Geometry: final body of the model. Coordinates: model frame, mm. A direction names the side the tool comes from. Give positions to 0.01 mm unless a question says otherwise; leave off trailing zeros. Order: outer loops, then holes, each group sorted by start corner. A loop starts at its lowest first (then second) coordinate and runs counter-clockwise, first axis right, second up. Notation, with made-up numbers: (-15.5, 85.25) -> (20.5, 85.25) arc R34 cw to (20.5, 119.25) -> close; hole circle Ø1 at (72, 30.25). An arc over 180 degrees is marked (long way). One line per question, with ' | ' between items. Start each with the question number.
(1) Section B-B (x = 60.5). Return loops of the section in (y, z).
(2) Mould query, pull axis Y, two halves, no side actions, for faces 6 (the face through (57, -23, 2)), 7 (the face through (35, -53, 5)), 8 (the face through (43.6, -91, -44.8)). Classes: +Y half, -Y half, draft (parallel to the pull), parting line (faces both ways), or undercut.
(3) First-contact query: pin 1 Ø1.5 at (x, z) = (46, -25.5) entering from +Y; pin 2 Ø12 at (y, z) = (-73.5, -6.5) entering from -X; pin 3 Ø6.5 at (x, y) = (60.5, -22.94) entering from -Z; pin 4 Ø13 at (x, z) = (40.5, -54) entering from +Y. Flat tips, straight axial feed; report the tip coordinate or a pass-through.
(4) Section D-D (z = -38.5). Return loops of the section in (x, y), then the cut area to 3 significant figures.
(5) Section A-A (z = -21.66). Return loops of the section in (x, y).
(6) Section C-C (y = -50). Return loops of the section in (x, z).
(7) Set-up query: faces 1 (the face through (43, -31.078, -21)), 2 (the face through (42, -27.878, -15)), 3 (the face through (44, -87.575, -54)), 4 (the face through (49.56, -53, -44)), 5 (the face through (43, -51, -46.5)). Return all of +Z, -Z, +X, -X, +Y, -Y with unobstructed straight access to the full face (end or side cutting, diameter ignored); none if empty.
(8) Ray query, L1, parallel to Y at x = 60.5, z = 3.6; L2, parallel to Z at x = 40, y = -69; L3, parallel to X at y = -74.5, z = -45. Return the intervals inside material, ascending.
```python
from build123d import *

# Parameters (mm, degrees)
BOSS_EXTRUDE1_DEPTH   = 5
SKETCH2_W             = 6.35
SKETCH2_H             = 50
BOSS_EXTRUDE2_DEPTH   = 52.48
CUT_EXTRUDE1_REACH    = 106.448
SKETCH3_R             = 20.44
SKETCH3_R_2           = 2.555
SKETCH3_W             = 5
SKETCH3_H             = 50
CUT_EXTRUDE2_REACH    = 108.104
SKETCH4_R             = 3.5
CUT_EXTRUDE6_REACH    = 108.104
SKETCH14_W            = 23.196263878
SKETCH14_H            = 15.316152196
SKETCH15_W            = 12
SKETCH15_H            = 3.2
BOSS_EXTRUDE7_DEPTH   = 46.5
BOSS_EXTRUDE8_REACH   = 98.667
SKETCH16_W            = 12
SKETCH16_H            = 3.5
SKETCH17_W            = 12
SKETCH17_H            = 3.5
BOSS_EXTRUDE9_DEPTH   = 15
CHAMFER2_SIZE         = 2
SKETCH22_W            = 12
SKETCH22_H            = 15
BOSS_EXTRUDE10_DEPTH  = 0.72
CUT_EXTRUDE8_REACH    = 103.606
CUT_EXTRUDE7_REACH    = 120.762
SKETCH18_R            = 3.25
MIRROR2_OUTLINE_W     = 50
MIRROR2_OUTLINE_H     = 5
MIRROR2_DEPTH         = 68
MIRROR2_2_OUTLINE_R   = 2.555
MIRROR2_2_OUTLINE_R_2 = 20.44
MIRROR2_2_DEPTH       = 6.35
MIRROR2_START         = 37.56
MIRROR2_3_DEPTH       = 12
MIRROR2_START_2       = 51
MIRROR2_4_OUTLINE_W   = 13.938985111
MIRROR2_4_OUTLINE_H   = 5
MIRROR2_4_DEPTH       = 5.9999999
MIRROR2_START_3       = 64.0000001
MIRROR2_5_OUTLINE_W   = 13.938985111
MIRROR2_5_OUTLINE_H   = 5
MIRROR2_5_DEPTH       = 5.9999999
MIRROR2_6_DEPTH       = 5
BOSS_EXTRUDE11_DEPTH  = 12
CUT_EXTRUDE9_REACH    = 132.799
SKETCH26_W            = 121.241742099
SKETCH26_H            = 103.992632166


with BuildPart() as part:
    # Sketch1 → Boss-Extrude1 (new body)
    with BuildSketch(Plane.XY):
        Polygon((0, 0), (0, 50), (51, 50), (51, 64.061014889), (70, 64.061014889), (70, -13.938985111), (51, -13.938985111), (51, 0), align=None)
    extrude(amount=BOSS_EXTRUDE1_DEPTH)

    # Sketch2 → Boss-Extrude2 (add)
    with BuildSketch(Plane(origin=(0, 0, 0), x_dir=(-1, 0, 0), z_dir=(0, 0, -1))):
        with Locations((-3.175, 25)):
            Rectangle(SKETCH2_W, SKETCH2_H)
    extrude(amount=BOSS_EXTRUDE2_DEPTH)

    # Sketch3 → Cut-Extrude1 (cut, up to next)
    with BuildSketch(Plane(origin=(6.35, 0, 0), x_dir=(0, 0, -1), z_dir=(1, 0, 0)), mode=Mode.PRIVATE) as cut_extrude1_sk1:
        with Locations((21.66, 25)):
            Circle(SKETCH3_R)
    cut_extrude1_tool1 = extrude(cut_extrude1_sk1.sketch, amount=-CUT_EXTRUDE1_REACH, mode=Mode.PRIVATE) & part.part
    # Sketch3 → Cut-Extrude1 (cut, up to next)
    with BuildSketch(Plane(origin=(6.35, 0, 0), x_dir=(0, 0, -1), z_dir=(1, 0, 0)), mode=Mode.PRIVATE) as cut_extrude1_sk2:
        with Locations((3.695, 42.955)):
            Circle(SKETCH3_R_2)
    cut_extrude1_tool2 = extrude(cut_extrude1_sk2.sketch, amount=-CUT_EXTRUDE1_REACH, mode=Mode.PRIVATE) & part.part
    # Sketch3 → Cut-Extrude1 (cut, up to next)
    with BuildSketch(Plane(origin=(6.35, 0, 0), x_dir=(0, 0, -1), z_dir=(1, 0, 0)), mode=Mode.PRIVATE) as cut_extrude1_sk3:
        with Locations((39.615, 7.045)):
            Circle(SKETCH3_R_2)
    cut_extrude1_tool3 = extrude(cut_extrude1_sk3.sketch, amount=-CUT_EXTRUDE1_REACH, mode=Mode.PRIVATE) & part.part
    # Sketch3 → Cut-Extrude1 (cut, up to next)
    with BuildSketch(Plane(origin=(6.35, 0, 0), x_dir=(0, 0, -1), z_dir=(1, 0, 0)), mode=Mode.PRIVATE) as cut_extrude1_sk4:
        with Locations((49.98, 25)):
            Rectangle(SKETCH3_W, SKETCH3_H)
    cut_extrude1_tool4 = extrude(cut_extrude1_sk4.sketch, amount=-CUT_EXTRUDE1_REACH, mode=Mode.PRIVATE) & part.part
    add(cut_extrude1_tool1.solids().sort_by_distance((6.35, 25, -21.66))[0], mode=Mode.SUBTRACT)
    add(cut_extrude1_tool2.solids().sort_by_distance((6.35, 42.955, -3.695))[0], mode=Mode.SUBTRACT)
    add(cut_extrude1_tool3.solids().sort_by_distance((6.35, 7.045, -39.615))[0], mode=Mode.SUBTRACT)
    add(cut_extrude1_tool4.solids().sort_by_distance((6.35, 25, -49.98))[0], mode=Mode.SUBTRACT)

    # Sketch4 → Cut-Extrude2 (cut, up to next)
    with BuildSketch(Plane(origin=(0, 0, 0), x_dir=(-1, 0, 0), z_dir=(0, 0, -1)), mode=Mode.PRIVATE) as cut_extrude2_sk1:
        with Locations((-60.5, 55.061014889)):
            Circle(SKETCH4_R)
    cut_extrude2_tool1 = extrude(cut_extrude2_sk1.sketch, amount=-CUT_EXTRUDE2_REACH, mode=Mode.PRIVATE) & part.part
    # Sketch4 → Cut-Extrude2 (cut, up to next)
    with BuildSketch(Plane(origin=(0, 0, 0), x_dir=(-1, 0, 0), z_dir=(0, 0, -1)), mode=Mode.PRIVATE) as cut_extrude2_sk2:
        with Locations((-60.5, -4.938985111)):
            Circle(SKETCH4_R)
    cut_extrude2_tool2 = extrude(cut_extrude2_sk2.sketch, amount=-CUT_EXTRUDE2_REACH, mode=Mode.PRIVATE) & part.part
    add(cut_extrude2_tool1.solids().sort_by_distance((60.5, 55.061015, 0))[0], mode=Mode.SUBTRACT)
    add(cut_extrude2_tool2.solids().sort_by_distance((60.5, -4.938985, 0))[0], mode=Mode.SUBTRACT)

    # Sketch14 → Cut-Extrude6 (cut, up to next)
    with BuildSketch(Plane(origin=(0, 0, 0), x_dir=(-1, 0, 0), z_dir=(0, 0, -1)), mode=Mode.PRIVATE) as cut_extrude6_sk1:
        with Locations((-62.598131939, 57.658076098)):
            Rectangle(SKETCH14_W, SKETCH14_H)
    cut_extrude6_tool1 = extrude(cut_extrude6_sk1.sketch, amount=-CUT_EXTRUDE6_REACH, mode=Mode.PRIVATE) & part.part
    add(cut_extrude6_tool1.solids().sort_by_distance((62.598132, 57.658076, 0))[0], mode=Mode.SUBTRACT)

    # Sketch15 → Boss-Extrude7 (add)
    with BuildSketch(Plane(origin=(0, 0, 0), x_dir=(-1, 0, 0), z_dir=(0, 0, -1))):
        with Locations((-43.56, 1.6)):
            Rectangle(SKETCH15_W, SKETCH15_H)
    extrude(amount=BOSS_EXTRUDE7_DEPTH)

    # Boss-Extrude8: up to this plane
    boss_extrude8_end = Plane(origin=(166.832994776, 64.085435133, -66.619565524), z_dir=(-1.1416993347548052e-15, 0.9990256874715413, 0.04413247978546202))
    # Sketch16 → Boss-Extrude8 (add, up to the surface)
    with BuildSketch(Plane(origin=(0, 3.2, 0), x_dir=(1, 0, 0), z_dir=(0, 1, 0)), mode=Mode.PRIVATE) as boss_extrude8_sk1:
        with Locations((43.56, 44.75)):
            Rectangle(SKETCH16_W, SKETCH16_H)
    boss_extrude8_tool1 = split(extrude(boss_extrude8_sk1.sketch, amount=BOSS_EXTRUDE8_REACH, mode=Mode.PRIVATE), bisect_by=boss_extrude8_end, keep=Keep.BOTH, mode=Mode.PRIVATE)
    add(boss_extrude8_tool1.solids().sort_by_distance((43.56, 3.2, -44.75))[0])

    # Sketch17 → Boss-Extrude9 (add)
    with BuildSketch(Plane(origin=(0, 0, -46.5), x_dir=(-1, 0, 0), z_dir=(0, 0, -1))):
        with Locations((-43.56, 61.446642853)):
            Rectangle(SKETCH17_W, SKETCH17_H)
    extrude(amount=BOSS_EXTRUDE9_DEPTH)

    # Chamfer2
    chamfer2_edges = [part.edges().sort_by_distance(p)[0] for p in [
        (3.175, 0, -47.48),
        (3.175, 50, -47.48),
        (70, 50, 2.5),
    ]]
    chamfer(chamfer2_edges, length=CHAMFER2_SIZE)

    # Sketch22 → Boss-Extrude10 (add)
    with BuildSketch(Plane(origin=(0, 63.196642853, 0), x_dir=(1, 0, 0), z_dir=(0, 1, 0))):
        with Locations((43.56, 54)):
            Rectangle(SKETCH22_W, SKETCH22_H)
    extrude(amount=BOSS_EXTRUDE10_DEPTH)

    # Sketch23 → Cut-Extrude8 (cut, up to next)
    with BuildSketch(Plane(origin=(49.56, 0, 0), x_dir=(0, 0, -1), z_dir=(1, 0, 0)), mode=Mode.PRIVATE) as cut_extrude8_sk1:
        Polygon((46.5, 63.916642853), (46.5, 63.196642853), (61.5, 63.916642853), align=None)
    cut_extrude8_tool1 = extrude(cut_extrude8_sk1.sketch, amount=-CUT_EXTRUDE8_REACH, mode=Mode.PRIVATE) & part.part
    add(cut_extrude8_tool1.solids().sort_by_distance((49.56, 63.676643, -51.5))[0], mode=Mode.SUBTRACT)

    # Cut-Extrude7: up to this plane
    cut_extrude7_end = Plane(origin=(-0.001, 63.196642853, -46.5), z_dir=(-2.1659106514416256e-15, -0.9988499868416298, -0.04794479936839813))
    # Sketch18 → Cut-Extrude7 (cut, up to the surface)
    with BuildSketch(Plane.XZ.offset(-59.696642853), mode=Mode.PRIVATE) as cut_extrude7_sk1:
        with Locations(Location((43.56, -52.57, 0), (0, 0, 270))):
            Circle(SKETCH18_R)
    cut_extrude7_tool1 = split(extrude(cut_extrude7_sk1.sketch, amount=-CUT_EXTRUDE7_REACH, mode=Mode.PRIVATE), bisect_by=cut_extrude7_end, keep=Keep.BOTH, mode=Mode.PRIVATE)
    add(cut_extrude7_tool1.solids().sort_by_distance((43.56, 59.696643, -52.57))[0], mode=Mode.SUBTRACT)



with BuildPart() as body_2:
    # Mirror2: read off the stored shape, not the designer's step
    # Mirror2 outline → Mirror2 (new body)
    with BuildSketch(Plane.YZ):
        with Locations((-52.877970222, 2.5)):
            Rectangle(MIRROR2_OUTLINE_W, MIRROR2_OUTLINE_H)
    extrude(amount=MIRROR2_DEPTH)

    # Mirror2 2 outline → Mirror2 2 (add)
    with BuildSketch(Plane.YZ):
        Polygon((-27.877970222, -45.48), (-27.877970222, 0), (-77.877970222, 0), (-77.877970222, -45.48), (-75.877970222, -47.48), (-29.877970222, -47.48), align=None)
        with Locations((-34.922970222, -39.615)):
            Circle(MIRROR2_2_OUTLINE_R, mode=Mode.SUBTRACT)
        with Locations((-70.832970222, -3.695)):
            Circle(MIRROR2_2_OUTLINE_R, mode=Mode.SUBTRACT)
        with Locations((-52.877970222, -21.66)):
            Circle(MIRROR2_2_OUTLINE_R_2, mode=Mode.SUBTRACT)
    extrude(amount=MIRROR2_2_DEPTH)


with BuildPart() as part_1:
    add(part.part)

    add(body_2.part)  # Mirror2 3 merges body 2
    # Mirror2 3 outline → Mirror2 3 (add)
    with BuildSketch(Plane.YZ.offset(MIRROR2_START)):
        Polygon((-31.077970222, -46.5), (0, -46.5), (0, -43), (-27.877970222, -43), (-27.877970222, 0), (-31.077970222, 0), align=None)
    extrude(amount=MIRROR2_3_DEPTH)

    # Mirror2 4 outline → Mirror2 4 (add)
    with BuildSketch(Plane.YZ.offset(MIRROR2_START_2)):
        with Locations((-20.908477667, 2.5)):
            Rectangle(MIRROR2_4_OUTLINE_W, MIRROR2_4_OUTLINE_H)
    extrude(amount=MIRROR2_4_DEPTH)

    # Mirror2 5 outline → Mirror2 5 (add)
    with BuildSketch(Plane.YZ.offset(MIRROR2_START_3)):
        with Locations((-20.908477667, 2.5)):
            Rectangle(MIRROR2_5_OUTLINE_W, MIRROR2_5_OUTLINE_H)
    extrude(amount=MIRROR2_5_DEPTH)

    # Mirror2 6 outline → Mirror2 6 (add)
    with BuildSketch(Plane.XY):
        Polygon((70, -75.877970222), (70, -27.877970222), (68, -27.877970222), (68, -77.877970222), align=None)
        with BuildLine():
            Line((64.0000001, -27.877970222), (64, -22.938985111))
            ThreePointArc((64, -22.938985111), (60.5, -26.438985111), (57, -22.938985111))
            Line((57, -22.938985111), (56.9999999, -27.877970222))
            Line((56.9999999, -27.877970222), (64.0000001, -27.877970222))
        make_face()
        with BuildLine():
            ThreePointArc((57, -22.938985111), (60.5, -19.438985111), (64, -22.938985111))
            Line((64, -22.938985111), (64.0000001, -13.938985111))
            Line((64.0000001, -13.938985111), (56.9999999, -13.938985111))
            Line((56.9999999, -13.938985111), (57, -22.938985111))
        make_face()
    extrude(amount=MIRROR2_6_DEPTH)

    # Sketch25 → Boss-Extrude11 (add)
    with BuildSketch(Plane(origin=(49.56, 0, 0), x_dir=(0, 0, -1), z_dir=(1, 0, 0))):
        Polygon((43, -13.938985111), (46.5, -13.938985111), (46.5, -87.574613075), (61.5, -87.574613075), (61.5, -91.794613075), (46.5, -91.074613075), (43, -90.919998753), (43, -31.077970222), align=None)
    extrude(amount=-BOSS_EXTRUDE11_DEPTH)

    # Cut-Extrude9: up to this face of the body (flat: up to its plane)
    cut_extrude9_end = Plane(part_1.part.faces().sort_by_distance((0, 0.724855186, -20.24))[0])
    # Sketch26 → Cut-Extrude9 (cut, up to the picked face)
    with BuildSketch(Plane(origin=(70, 0, 0), x_dir=(0, 0, -1), z_dir=(1, 0, 0)), mode=Mode.PRIVATE) as cut_extrude9_sk1:
        with Locations((55.62087105, 38.057330972)):
            Rectangle(SKETCH26_W, SKETCH26_H)
    cut_extrude9_tool1 = split(extrude(cut_extrude9_sk1.sketch, amount=-CUT_EXTRUDE9_REACH, mode=Mode.PRIVATE), bisect_by=cut_extrude9_end, keep=Keep.BOTH, mode=Mode.PRIVATE)
    add(cut_extrude9_tool1.solids().sort_by(Axis((70, 38.057331, -55.620871), (-1, 0, 0)))[0], mode=Mode.SUBTRACT)


solid = part_1.part
```
Response:
1) outline: (-77.88, 0) -> (-26.44, 0) -> (-26.44, 5) -> (-77.88, 5) -> close; (-19.44, 0) -> (-13.94, 0) -> (-13.94, 5) -> (-19.44, 5) -> close
2) face 6: undercut | face 7: draft | face 8: -Y half
3) pin 1: stops at y = -27.88 | pin 2: stops at x = 0 | pin 3: passes through | pin 4: stops at y = -87.57
4) outline: (0, -77.88) -> (6.35, -77.88) -> (6.35, -64.46) -> (0, -64.46) -> close; (0, -41.29) -> (6.35, -41.29) -> (6.35, -37.22) -> (0, -37.22) -> close; (0, -32.62) -> (6.35, -32.62) -> (6.35, -27.88) -> (0, -27.88) -> close; (37.56, -31.08) -> (49.56, -31.08) -> (49.56, -27.88) -> (37.56, -27.88) -> close | area: 180 mm^2
5) outline: (0, -77.88) -> (6.35, -77.88) -> (6.35, -73.32) -> (0, -73.32) -> close; (0, -32.44) -> (6.35, -32.44) -> (6.35, -27.88) -> (0, -27.88) -> close; (37.56, -31.08) -> (49.56, -31.08) -> (49.56, -27.88) -> (37.56, -27.88) -> close
6) outline: (0, -47.48) -> (6.35, -47.48) -> (6.35, -41.9) -> (0, -41.9) -> close; (0, -1.42) -> (6.35, -1.42) -> (6.35, 0) -> (70, 0) -> (70, 5) -> (0, 5) -> close; (37.56, -46.5) -> (49.56, -46.5) -> (49.56, -43) -> (37.56, -43) -> close
7) face 1: +X, -Y | face 2: +Z, -X, +Y | face 3: -Z, +X, -X, +Y | face 4: -Z, +X, +Y, -Y | face 5: -Z, +X, +Y
8) L1: y = -77.88 to -26.44, -19.44 to -13.94 | L2: z = -46.5 to -43, 0 to 5 | L3: x = 0 to 6.35, 37.56 to 49.56
